```python
from build123d import *

# Parameters (mm, degrees)
SKETCH1_R           = 2.35
BOSS_EXTRUDE1_DEPTH = 3
FILLET1_R           = 3
FILLET2_R           = 1


with BuildPart() as part:
    # Sketch1 → Boss-Extrude1 (new body)
    with BuildSketch(Plane(origin=(0, 0, 0), x_dir=(1, 0, 0), z_dir=(0, 1, 0))):
        with BuildLine():
            Line((172.530209002, -85.760018057), (151.631467282, -106.990912204))
            ThreePointArc((151.631467282, -106.990912204), (145.936608589, -106.997416648), (146.006888843, -101.302987922))
            Line((146.006888843, -101.302987922), (166.487269252, -81.589717624))
            Line((166.487269252, -81.589717624), (159.587325171, -70.634585049))
            ThreePointArc((159.587325171, -70.634585049), (161.101414603, -60.775325043), (158.208232615, -70.321369913))
            Line((158.208232615, -70.321369913), (110.989592357, -100.061400455))
            ThreePointArc((110.989592357, -100.061400455), (103.665172589, -106.143163876), (99.686339562, -97.494241459))
            Line((99.686339562, -97.494241459), (98.064605927, -94.919393494))
            Line((98.064605927, -94.919393494), (91.923450353, -94.919393494))
            Line((91.923450353, -94.919393494), (90.301716718, -97.494241459))
            ThreePointArc((90.301716718, -97.494241459), (86.322883691, -106.143163876), (78.998463923, -100.061400455))
            Line((78.998463923, -100.061400455), (31.779823665, -70.321369913))
            ThreePointArc((31.779823665, -70.321369913), (28.886641677, -60.775325043), (30.400731109, -70.634585049))
            Line((30.400731109, -70.634585049), (24.422488643, -80.126319765))
            Line((24.422488643, -80.126319765), (23.686968876, -83.726197894))
            ThreePointArc((23.686968876, -83.726197894), (18.589619222, -86.469487176), (16.804675386, -80.962892486))
            Line((16.804675386, -80.962892486), (24.563909918, -68.643453086))
            ThreePointArc((24.563909918, -68.643453086), (28.620869821, -59.605126205), (36.183956221, -66.00434495))
            Line((36.183956221, -66.00434495), (83.208225156, -95.621953308))
            ThreePointArc((83.208225156, -95.621953308), (86.101407144, -105.167998178), (84.587317712, -95.308738171))
            Line((84.587317712, -95.308738171), (89.761234685, -87.094041689))
            Line((89.761234685, -87.094041689), (90.99402814, -82.971663764))
            ThreePointArc((90.99402814, -82.971663764), (94.99402814, -78.971663764), (98.99402814, -82.971663764))
            Line((98.99402814, -82.971663764), (100.212762732, -87.071720247))
            Line((100.212762732, -87.071720247), (105.400738568, -95.308738171))
            ThreePointArc((105.400738568, -95.308738171), (103.886649136, -105.167998178), (106.779831124, -95.621953308))
            Line((106.779831124, -95.621953308), (153.804100058, -66.00434495))
            ThreePointArc((153.804100058, -66.00434495), (161.367186459, -59.605126205), (165.424146361, -68.643453086))
            Line((165.424146361, -68.643453086), (173.183380893, -80.962892486))
            ThreePointArc((173.183380893, -80.962892486), (173.728802193, -83.480186919), (172.530209002, -85.760018057))
        make_face()
        with Locations((148.780829272, -104.184871767)):
            Circle(SKETCH1_R, mode=Mode.SUBTRACT)
        Polygon((167.74402814, -82.071663764), (167.74402814, -83.871663764), (169.09402814, -83.871663764), (169.09402814, -85.221663764), (170.89402814, -85.221663764), (170.89402814, -83.871663764), (172.24402814, -83.871663764), (172.24402814, -82.071663764), (170.89402814, -82.071663764), (170.89402814, -80.721663764), (169.09402814, -80.721663764), (169.09402814, -82.071663764), align=None, mode=Mode.SUBTRACT)
        Polygon((92.74402814, -82.071663764), (92.74402814, -83.871663764), (94.09402814, -83.871663764), (94.09402814, -85.221663764), (95.89402814, -85.221663764), (95.89402814, -83.871663764), (97.24402814, -83.871663764), (97.24402814, -82.071663764), (95.89402814, -82.071663764), (95.89402814, -80.721663764), (94.09402814, -80.721663764), (94.09402814, -82.071663764), align=None, mode=Mode.SUBTRACT)
        Polygon((17.74402814, -82.071663764), (17.74402814, -83.871663764), (19.09402814, -83.871663764), (19.09402814, -85.221663764), (20.89402814, -85.221663764), (20.89402814, -83.871663764), (22.24402814, -83.871663764), (22.24402814, -82.071663764), (20.89402814, -82.071663764), (20.89402814, -80.721663764), (19.09402814, -80.721663764), (19.09402814, -82.071663764), align=None, mode=Mode.SUBTRACT)
    extrude(amount=BOSS_EXTRUDE1_DEPTH)

    # Fillet1
    fillet1_edges = [part.edges().sort_by_distance(p)[0] for p in [
        (166.487269252, 1.5, 81.589717624),
        (159.587325171, 1.5, 70.634585049),
        (158.208232615, 1.5, 70.321369913),
        (31.779823665, 1.5, 70.321369913),
        (30.400731109, 1.5, 70.634585049),
        (83.208225156, 1.5, 95.621953308),
        (84.587317712, 1.5, 95.308738171),
        (105.400738568, 1.5, 95.308738171),
        (106.779831124, 1.5, 95.621953308),
    ]]
    fillet(fillet1_edges, radius=FILLET1_R)

    # Fillet2
    fillet2_edges = [part.edges().sort_by_distance(p)[0] for p in [
        (110.989592357, 1.5, 100.061400455),
        (99.686339562, 1.5, 97.494241459),
        (90.301716718, 1.5, 97.494241459),
        (78.998463923, 1.5, 100.061400455),
        (24.422488643, 1.5, 80.126319765),
        (24.563909918, 1.5, 68.643453086),
        (36.183956221, 1.5, 66.00434495),
        (89.761234685, 1.5, 87.094041689),
        (90.99402814, 1.5, 82.971663764),
        (98.99402814, 1.5, 82.971663764),
        (100.212762732, 1.5, 87.071720247),
        (153.804100058, 1.5, 66.00434495),
        (165.424146361, 1.5, 68.643453086),
    ]]
    fillet(fillet2_edges, radius=FILLET2_R)


solid = part.part
```
For this review, take the finished solid that the model builds, in its own axes (mm). A direction names the side the tool comes from. Coordinates: 2 decimals unless noted, no trailing zeros. Write each loop counter-clockwise with the first axis right and the second up, starting at its lowest first coordinate (ties: lowest second). Pieces come first, ordered by that corner, then holes.
(1) Add section A-A on z = 64. Give the boundary of the cut face in (x, y).
(2) Tool access review of faces 1 (the face through (101, 0, 89)), 2 (the face through (161.325, 1.521, 71.788)), 3 (the face through (101.757, 1.479, 89.523)), 4 (the face through (26.421, 1.479, 76.954)), 5 (the face through (173.734, 1.479, 83.444)): name each direction out of +Z, -Z, +X, -X, +Y, -Y from which nothing blocks a thin tool from reaching the whole face with its end or side.
(3) Wall thickness on probe 1 along X at (y, z) = (1.2, 90); probe 2 along X at (y, z) = (0.55, 65.5); probe 3 along X at (y, z) = (1.9, 99.5): over which ranges is each line inside the solid? List them lowest first.
(4) Add section D-D on x = 83.5. Give the boundary of the cut face in (y, z), then the cut area to 3 significant figures.
(5) Add section C-C on y = 0.55. Count the separate pieces of the cut face and the enclosed holes in it, then the cut area to 3 significant figures.
(6) For pin 1 Ø1.1 at (y, z) = (1, 81.5) entering from +X; pin 2 Ø0.7 at (y, z) = (1.5, 81) entering from -X; pin 3 Ø0.9 at (x, y) = (19.5, 1) entering from +Z, all flat-tipped, find the tip position at first contact; note any pin that passes through.
(7) The part is to be moulded in two halves that separate along Z. For faces 6 (the face through (24.04, 1.48, 81.99)), 7 (the face through (133.44, 1.48, 85.92)), 8 (the face through (101, 3, 89)), say which applies: +Z half, -Z half, draft (parallel to the pull), parting line (faces both ways), or undercut.
(8) Add section B-B on x = 50. Give the boundary of the cut face in (y, z).
Answer sheet:
1. outline: (24.02, 0) - (25.27, 0) - (25.27, 3) - (24.02, 3) - close; (34.71, 0) - (35.97, 0) - (35.97, 3) - (34.71, 3) - close; (154.02, 0) - (155.27, 0) - (155.27, 3) - (154.02, 3) - close; (164.71, 0) - (165.97, 0) - (165.97, 3) - (164.71, 3) - close
2. face 1: +Z, -Z, +X, -X, -Y
2. face 2: +Y, -Y
2. face 3: -Z, +Y, -Y
2. face 4: +Z, +Y, -Y
2. face 5: +X, +Y, -Y
3. probe 1: x = 63.02 to 74.28, 87.93 to 102.06, 115.71 to 126.96, 157.75 to 168.36
3. probe 2: x = 23.8 to 25, 34.99 to 36.19, 153.8 to 155, 164.99 to 166.19
3. probe 3: x = 78.11 to 80.06, 89.93 to 90.94, 99.05 to 100.06, 109.93 to 111.88, 147.88 to 159.01
4. outline: (0, 105.06) - (3, 105.06) - (3, 106.1) - (0, 106.1) - close
4. area: 3.12 mm2
5. separate pieces: 1
5. enclosed holes: 4
5. area: 1,350 mm2
6. pin 1: stops at x = 173.65
6. pin 2: stops at x = 16.59
6. pin 3: stops at z = 86.74
7. face 6: +Z half
7. face 7: undercut
7. face 8: draft
8. outline: (0, 74.71) - (3, 74.71) - (3, 81.8) - (0, 81.8) - close
